Part model, mm, in its own coordinate system. Face numbers are marked on the shaded views. A direction names the side the tool comes from. Round coordinates to 2 decimals unless told otherwise and drop trailing zeros. Write each loop counter-clockwise with the first axis right and the second up, starting at its lowest first coordinate (ties: lowest second). Pieces come first, ordered by that corner, then holes. Notation, with made-up numbers: (-38.75, 60) -> (-13.75, 60) arc R19 ccw to (-13.75, 65) -> close; hole circle Ø8 at (0.5, 44). An arc over 180 degrees is marked (long way). Use CSV: the item, a comma, the result in double quotes. Start each with the question number.
(1) Probe line 1 (Z direction, x = 1.2, y = 75.85); line 2 (X direction, y = 79.7, z = 2); line 3 (X direction, y = 48.5, z = 6.75). List the from-to ranges inside material, lowest first. Write a range as [from, to].
(2) Saw through at B-B (y = 10). Give the cut face in (x, z).
(3) Saw through at D-D (z = 7). Give the cut face in (x, y).
(4) Drop flat-ended pins along their axis: pin 1 (3 mm diameter, centred on x = 10.5, y = 18, fed in from +Z); pin 2 (6 mm diameter, centred on y = 76.5, z = 22, fed in from +X). Give the stop position or say it passes through.
(5) Saw through at C-C (x = 13.75). Give the cut face in (y, z).
(6) Which spindle directions (+Z, -Z, +X, -X, +Y, -Y) get a long thin tool onto all of the face, cutting with end or side? Do the marked faces 1 and 2. Say none if no direction does.
(7) Saw through at A-A (y = 75.85). Give the cut face in (x, z), plus the area to 3 significant figures.
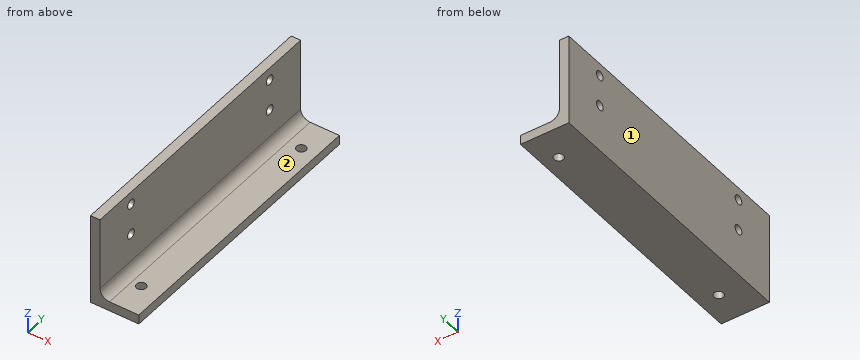
Autodesk Fusion 360 part; units mm, degrees
sketch "Sketch1" plane through (0, 0, 0) normal (0, 0, 1) x (1, 0, 0)
  line L0 (0, 0) -> (15.3, 0)
  line L1 (15.3, 0) -> (15.3, 89.7)
  line L2 (15.3, 89.7) -> (0, 89.7)
  line L3 (0, 89.7) -> (0, 0)
  circle A0 centre (9, 10) radius 1.5
  circle A1 centre (10.3, 79.7) radius 1.5
  dimension "d1" = 3
  dimension "d2" = 3
  dimension "d3" = 69.7
  dimension "d4" = 1.3
  dimension "d5" = 10
  dimension "d6" = 10
  dimension "d7" = 9
  dimension "d8" = 5
extrude "Extrude1" add sketch "Sketch1" along normal blind 3
sketch "Sketch2" plane through (0, 0, 3) normal (0, 0, 1) x (-1, 0, 0)
  circle A0 centre (-10.3, -79.7) radius 1.5
  circle A1 centre (-9, -10) radius 1.5
  line L0 (0, -89.7) -> (0, 0)
  line L1 (0, 0) -> (-15.3, 0)
  line L2 (-15.3, 0) -> (-15.3, -89.7)
  line L3 (-15.3, -89.7) -> (0, -89.7)
  line L4 (0, -89.7) -> (-3, -89.7)
  line L5 (-3, -89.7) -> (-3, 0)
  line L6 (-3, 0) -> (0, 0)
  line L7 (0, 0) -> (0, -89.7)
  dimension "d11" = 3
extrude "Extrude2" add sketch "Sketch2" along normal blind 26 contours L0 L1 L3 L4 L5 L6 L7
sketch "Sketch3" plane through (0, 0, 0) normal (-1, 0, 0) x (0, -1, 0)
  line L0 (-89.7, 0) -> (0, 0)
  line L1 (0, 0) -> (0, 29)
  line L2 (0, 29) -> (-89.7, 29)
  line L3 (-89.7, 29) -> (-89.7, 0)
  line L4 (-75.85, 25) -> (-13.85, 25) construction
  line L5 (-13.85, 25) -> (-13.85, 15) construction
  line L6 (-13.85, 15) -> (-75.85, 15) construction
  line L7 (-75.85, 15) -> (-75.85, 25) construction
  line L8 (-44.85, 29) -> (-44.85, 0) construction
  line L9 (-75.85, 20) -> (-13.85, 20) construction
  line L10 (-44.85, 25) -> (-44.85, 15) construction
  circle A0 centre (-75.85, 25) radius 1.5
  circle A1 centre (-13.85, 25) radius 1.5
  circle A2 centre (-13.85, 15) radius 1.5
  circle A3 centre (-75.85, 15) radius 1.5
  dimension "d14" = 62
  dimension "d15" = 10
  dimension "d16" = 4
  dimension "d17" = 3
  dimension "d18" = 3
  dimension "d19" = 3
  dimension "d20" = 3
extrude "Extrude3" cut sketch "Sketch3" against normal blind 20 contours A0 | A1 | A2 | A3
fillet "Fillet1" radius 3 1 edges at (3, 44.85, 3)
Answers:
1,line 1,"z = [0, 13.5], [16.5, 23.5], [26.5, 29]"
1,line 2,"x = [0, 8.8], [11.8, 15.3]"
1,line 3,"x = [0, 3]"
2,outline,"(0, 0) -> (7.5, 0) -> (7.5, 3) -> (6, 3) arc R3 cw to (3, 6) -> (3, 29) -> (0, 29) -> close; (10.5, 0) -> (15.3, 0) -> (15.3, 3) -> (10.5, 3) -> close"
3,outline,"(0, 0) -> (3, 0) -> (3, 89.7) -> (0, 89.7) -> close"
4,pin 1,"stops at z = 3"
4,pin 2,"stops at x = 3"
5,outline,"(0, 0) -> (89.7, 0) -> (89.7, 3) -> (0, 3) -> close"
6,face 1,"+Z, -Z, -X, +Y, -Y"
6,face 2,"+Z, +X, +Y, -Y"
7,outline,"(0, 0) -> (15.3, 0) -> (15.3, 3) -> (6, 3) arc R3 cw to (3, 6) -> (3, 13.5) -> (0, 13.5) -> close; (0, 16.5) -> (3, 16.5) -> (3, 23.5) -> (0, 23.5) -> close; (0, 26.5) -> (3, 26.5) -> (3, 29) -> (0, 29) -> close"
7,area,"108 mm²"
